Geometry: see drawing. Coordinates: mm, zero at the bounding-box minimum. A direction names the side the tool comes from. Give positions to 0.01 mm unless a question says otherwise; leave off trailing zeros. Order: outer loops, then holes, each group sorted by start corner. A loop starts at its lowest first (then second) coordinate and runs counter-clockwise, first axis right, second up. Notation, with made-up numbers: (32.5, -18) -> (39.5, -18) arc R32 ccw to (39.5, 19) -> close; hole circle Ø9 at (-1, 17). An arc over 180 degrees is marked (long way). One line per item, written item: value. Start each with the question number.
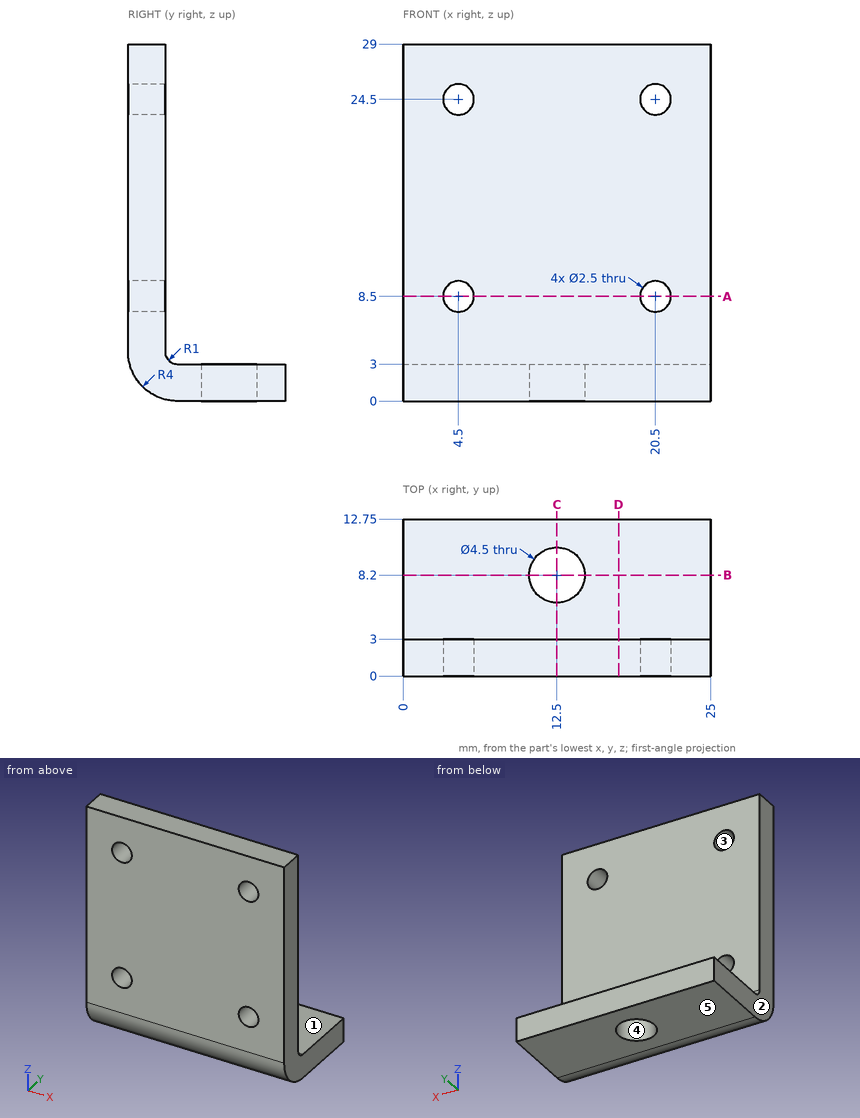
1. Cut plane D-D, the plane x = 17.5. Return loops of the section in (y, z).
2. Cut plane B-B, the plane y = 8.2. Return loops of the section in (x, z).
3. Material intervals for L1, parallel to X at y = 2.05, z = 24.5; L2, parallel to Z at x = 4.5, y = 0.9; L3, parallel to Z at x = 20.5, y = 1.2, sorted ascending. Write a range as [from, to].
4. Access query for the marked faces 1 and 2. Directions: +Z, -Z, +X, -X, +Y, -Y. A direction counts if a zero-diameter tool reaches every point of the face in a straight line with its end or side. Return the directions, or none.
5. Draft query along Z for the marked faces 3, 4 and 5. Return one class per face: pulls with the +Z half, pulls with the -Z half, needs draft (parallel to the pull), parting line crosses it, or undercut.
6. Cut plane A-A, the plane z = 8.5. Return loops of the section in (x, y), then the cut area to 3 significant figures.
7. Pin query (flat end, axial travel): P1, Ø4, axis at x = 20.5, z = 24.5, coming from the +Y side; P2, Ø5, axis at x = 3.5, y = 7.5, coming from the +Z side; P3, Ø4, axis at x = 12.5, y = 8.2, coming from the -Z side; P4, Ø3, axis at x = 14, y = 5, coming from the +Z side. Return the tip coordinate at first contact, or that it passes through.
8. Cut plane C-C, the plane x = 12.5. Return loops of the section in (y, z), then the cut area to 3 significant figures.
Answers follow:
1. outline: (0, 4) arc R4 ccw to (4, 0) -> (12.75, 0) -> (12.75, 3) -> (4, 3) arc R1 cw to (3, 4) -> (3, 29) -> (0, 29) -> close
2. outline: (0, 0) -> (10.25, 0) -> (10.25, 3) -> (0, 3) -> close; (14.75, 0) -> (25, 0) -> (25, 3) -> (14.75, 3) -> close
3. L1: x = [0, 3.25], [5.75, 19.25], [21.75, 25]
3. L2: z = [1.47, 7.25], [9.75, 23.25], [25.75, 29]
3. L3: z = [1.14, 7.25], [9.75, 23.25], [25.75, 29]
4. face 1: +Z, +X, -X, +Y
4. face 2: +Z, -Z, -X, +Y, -Y
5. face 3: undercut
5. face 4: needs draft
5. face 5: pulls with the -Z half
6. outline: (0, 0) -> (3.25, 0) -> (3.25, 3) -> (0, 3) -> close; (5.75, 0) -> (19.25, 0) -> (19.25, 3) -> (5.75, 3) -> close; (21.75, 0) -> (25, 0) -> (25, 3) -> (21.75, 3) -> close
6. area: 60.0 mm²
7. P1: stops at y = 3
7. P2: stops at z = 3
7. P3: passes through
7. P4: stops at z = 3.13
8. outline: (0, 4) arc R4 ccw to (4, 0) -> (5.95, 0) -> (5.95, 3) -> (4, 3) arc R1 cw to (3, 4) -> (3, 29) -> (0, 29) -> close; (10.45, 0) -> (12.75, 0) -> (12.75, 3) -> (10.45, 3) -> close
8. area: 99.5 mm²
